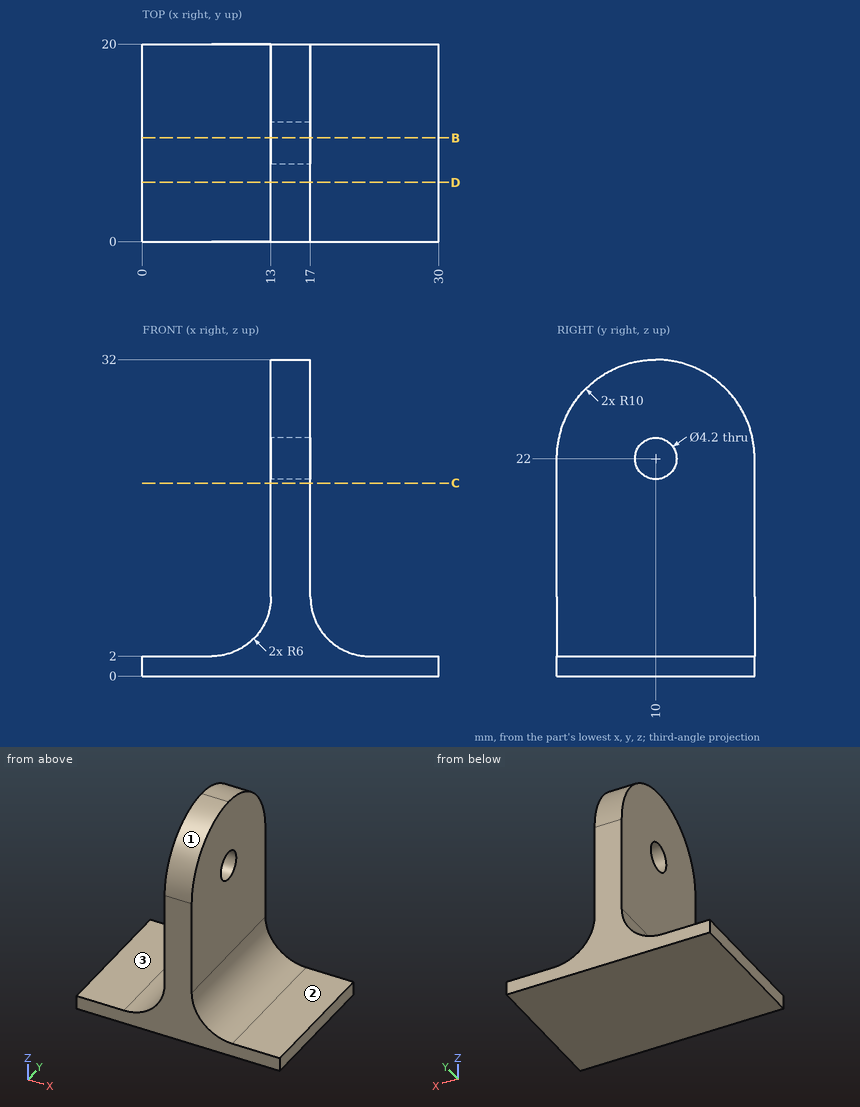
Study the drawing (mm; zero at the part's minimum x, y, z) and answer. A direction names the side the tool comes from. Give positions to 0.01 mm unless a question says otherwise; leave off trailing zeros. Write each loop counter-clockwise with the first axis right and the second up, starting at its lowest first coordinate (ties: lowest second). Pieces come first, ordered by that corner, then holes. Notation, with made-up numbers: (62, 46) - (82, 46) arc R21 cw to (82, 51) - close; hole circle Ø10 at (-21.75, 19). An arc over 180 degrees is marked (long way). Write item = value, one per line. Start each with the question number.
Item 1: Find section D-D (y = 6). Give the vertices of the cut face in (x, z) (3 decimals).
Item 2: Find section B-B (y = 10.5). Give the vertices of the cut face in (x, z), then the cut area to 3 significant figures.
Item 3: Find the intervals of material crossed by probe 1 along Z at (x, y) = (15.8, 10); probe 2 along X at (y, z) = (15, 13); probe 3 along Z at (x, y) = (3.5, 9.5), in increasing order. Write a range as [from, to].
Item 4: Find section C-C (z = 19.5). Give the vertices of the cut face in (x, y).
Item 5: Each of these flat-tipped pins is pushed along its axis until it touches: P1, Ø12, axis at y = 8.5, z = 14.5, coming from the -X side; P2, Ø3.5, axis at x = 27.5, y = 9, coming from the +Z side; P3, Ø4, axis at x = 6.5, y = 4, coming from the +Z side; P4, Ø10, axis at x = 8.5, y = 3.5, coming from the -Z side. Where does it stop, or does it pass through?
Item 6: A tool of negligible diameter and unlimited length cuts with its end or side. For the marked faces 1, 2 and 3, from which of +Z, -Z, +X, -X, +Y, -Y can it reach the whole face along a straight path? Write none if from no direction.
Response:
q1.outline = (0, 0) - (30, 0) - (30, 2) - (23, 2) arc R6 cw to (17, 8) - (17, 31.165) - (13, 31.165) - (13, 8) arc R6 cw to (7, 2) - (0, 2) - close
q2.outline = (0, 0) - (30, 0) - (30, 2) - (23, 2) arc R6 cw to (17, 8) - (17, 19.96) - (13, 19.96) - (13, 8) arc R6 cw to (7, 2) - (0, 2) - close; (13, 24.04) - (17, 24.04) - (17, 31.99) - (13, 31.99) - close
q2.area = 179 mm²
q3.probe_1 = [0, 19.9], [24.1, 32]
q3.probe_2 = [13, 17]
q3.probe_3 = [0, 2]
q4.outline = (13, 0) - (17, 0) - (17, 20) - (13, 20) - close
q5.P1 = 13
q5.P2 = 2
q5.P3 = 2.19
q5.P4 = 0
q6.face_1 = +Z, +X, -X, -Y
q6.face_2 = +Z, +X, +Y, -Y
q6.face_3 = +Z, -X, +Y, -Y
